Part model, mm, in its own coordinate system. Face numbers are marked on the shaded views. A direction names the side the tool comes from. Give positions to 0.01 mm unless a question says otherwise; leave off trailing zeros. Write each loop counter-clockwise with the first axis right and the second up, starting at its lowest first coordinate (ties: lowest second). Pieces come first, ordered by that corner, then holes.
from build123d import *

# Parameters (mm, degrees)
RECTANGLE001_W   = 128
RECTANGLE001_H   = 38
EXTRUDE001_DEPTH = 124
RECTANGLE_W      = 130
RECTANGLE_H      = 40
EXTRUDE_DEPTH    = 120


with BuildPart() as extrude001:
    # Rectangle001 → Extrude001 (new body)
    with BuildSketch(Plane(origin=(65, -2, 20), x_dir=(1, 0, 0), z_dir=(0, 1, 0))):
        Rectangle(RECTANGLE001_W, RECTANGLE001_H)
    extrude(amount=EXTRUDE001_DEPTH)


with BuildPart() as cut:
    # Rectangle → Extrude (new body)
    with BuildSketch(Plane(origin=(65, 0, 20), x_dir=(1, 0, 0), z_dir=(0, 1, 0))):
        Rectangle(RECTANGLE_W, RECTANGLE_H)
    extrude(amount=EXTRUDE_DEPTH)

    # Cut: cut Extrude001
    add(extrude001.part, mode=Mode.SUBTRACT)


solid = cut.part
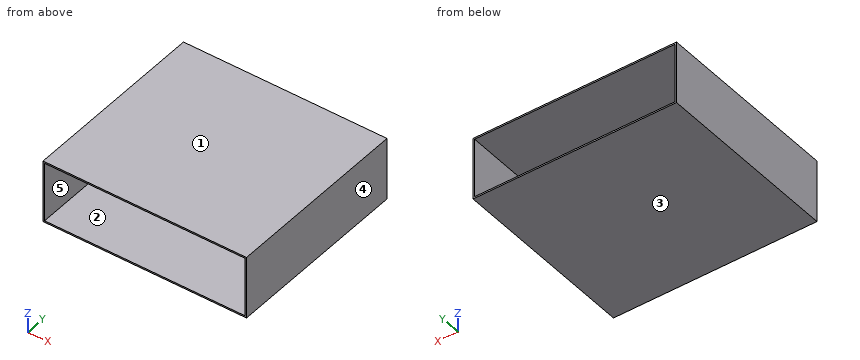
1) Saw through at C-C (z = 8.5). Write the cut outline in (x, y).
Check result:
outline: (0, 0) - (1, 0) - (1, 120) - (0, 120) - close; (129, 0) - (130, 0) - (130, 120) - (129, 120) - close
2) Mould opens along Z. For the marked faces 1, 2 and 3 say: +Z half, -Z half, draft (parallel to the pull), parting line (faces both ways), or undercut.
Check result:
face 1: +Z half
face 2: undercut
face 3: -Z half
3) 3-axis set-ups, long thin cutter, end or side, ignore diameter. For the marked faces 4 and 5: which of +Z, -Z, +X, -X, +Y, -Y reach the whole face in a straight line?
Check result:
face 4: +Z, -Z, +X, +Y, -Y
face 5: +Y, -Y
4) Saw through at A-A (y = 92). Write the cut outline in (x, z).
Check result:
outline: (0, 0) - (130, 0) - (130, 40) - (0, 40) - close; hole (1, 1) - (129, 1) - (129, 39) - (1, 39) - close
5) Drill centre lines: L1, parallel to X at y = 77, z = 7.5; L2, parallel to Z at x = 112.5, y = 44. Where is each one in solid material? Low to high.
Check result:
L1: x = 0 to 1, 129 to 130
L2: z = 0 to 1, 39 to 40
6) Saw through at B-B (x = 56). Write the cut outline in (y, z).
Check result:
outline: (0, 0) - (120, 0) - (120, 1) - (0, 1) - close; (0, 39) - (120, 39) - (120, 40) - (0, 40) - close
